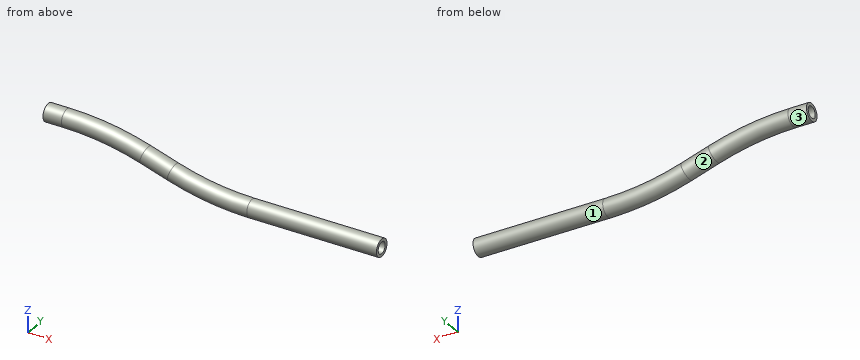
from build123d import *

# Parameters (mm, degrees)
F0_R   = 3
F0_R_2 = 2


with BuildPart() as f2:
    # F2: sweep along a path in F1
    with BuildLine(Plane.XZ) as f2_path:
        Line((0, 0), (-44.45, 0))
        ThreePointArc((-44.45, 0), (-58.1253747721, 1.0581300014), (-71.4752079395, 4.2073312746))
        Line((-71.4752079395, 4.2073312746), (-80.9247920605, 7.2226687254))
        ThreePointArc((-80.9247920605, 7.2226687254), (-94.2746252279, 10.3718699986), (-107.95, 11.43))
        Line((-107.95, 11.43), (-114.3, 11.43))
    # F0 (on Right) → F2 (sweep)
    with BuildSketch(Plane.YZ):
        Circle(F0_R)
        Circle(F0_R_2, mode=Mode.SUBTRACT)
    sweep(path=f2_path.line)


solid = f2.part
Check sheet for the modelled part. Datum: model origin and axes. Units: mm. Face numbers are marked on the shaded views. A direction names the side the tool comes from. Round coordinates to 2 decimals unless told otherwise and drop trailing zeros. Loops run counter-clockwise (first coordinate to the right, second up) from the corner with the lowest first, then second, coordinate; pieces in that order, holes last. Notation, with made-up numbers: (-20.75, 87.25) -> (7.25, 87.25) arc R36 cw to (7.25, 126.25) -> close; hole circle Ø5 at (61, 54.5). An arc over 180 degrees is marked (long way). Put each result on its own line as item: value. Start each with the question number.
1. Section check B-B (x = -39). Enter the section's corners in (y, z), plus the area to 3 significant figures.
2. Scan lines: probe 1 along Z at (x, y) = (-34, 0); probe 2 along Z at (x, y) = (-112.5, 0). Record each from-to range of solid material in increasing order.
3. Access from +Z, -Z, +X, -X, +Y, -Y to the whole of each face (thin tool, end or side, straight path). Record for the marked faces 1, 2 and 3.
4. Gauge pin test, flat ends, axial feed: pin 1 (1.5 mm diameter, centred on x = -35, z = 4, fed in from +Y); pin 2 (3 mm diameter, centred on x = -73.5, y = 2, fed in from -Z); pin 3 (1 mm diameter, centred on x = -24.5, y = -1.5, fed in from +Z). Record the tip position at first contact, or that the pin passes through.
5. Section check A-A (y = 0). Enter the section's corners in (x, z), plus the area to 3 significant figures.
Findings:
1. outline: circle Ø6 at (0, 0); hole circle Ø4 at (0, 0)
1. area: 15.7 mm^2
2. probe 1: z = -3 to -2, 2 to 3
2. probe 2: z = 8.43 to 9.43, 13.43 to 14.43
3. face 1: +X
3. face 2: none
3. face 3: -X
4. pin 1: passes through
4. pin 2: stops at z = 1.52
4. pin 3: stops at z = 2.83
5. outline: (-114.3, 8.43) -> (-107.95, 8.43) arc R85.9 cw to (-81.84, 4.36) -> (-72.39, 1.35) arc R91.9 ccw to (-44.45, -3) -> (0, -3) -> (0, -2) -> (-44.45, -2) arc R90.9 cw to (-72.08, 2.3) -> (-81.53, 5.32) arc R86.9 ccw to (-107.95, 9.43) -> (-114.3, 9.43) -> close; (-114.3, 13.43) -> (-107.95, 13.43) arc R90.9 cw to (-80.32, 9.13) -> (-70.87, 6.11) arc R86.9 ccw to (-44.45, 2) -> (0, 2) -> (0, 3) -> (-44.45, 3) arc R85.9 cw to (-70.56, 7.07) -> (-80.01, 10.08) arc R91.9 ccw to (-107.95, 14.43) -> (-114.3, 14.43) -> close
5. area: 231 mm^2
